from build123d import *

# Parameters (mm, degrees)
CYLINDER002_R         = 3.5
CYLINDER002_DEPTH     = 10
CYLINDER001_R         = 1.5
CYLINDER001_DEPTH     = 10
FUSION001_PITCH_ANGLE = 90
ARRAY001_COUNT        = 4
BOX002_W              = 6
BOX002_H              = 40
BOX002_DEPTH          = 25
CYLINDER_R            = 1.725
CYLINDER_DEPTH        = 10
ARRAY_X_COUNT         = 6
ARRAY_X_PITCH         = 20.333333
BOX_W                 = 194
BOX_H                 = 10
BOX_DEPTH             = 10
CHAMFER_SIZE          = 5


with BuildPart() as cylinder002:
    # Cylinder002 → Cylinder002 (new body)
    with BuildSketch(Plane(origin=(15, -5, 8), x_dir=(1, 0, 0), z_dir=(0, 0, 1))):
        Circle(CYLINDER002_R)
    extrude(amount=CYLINDER002_DEPTH)


with BuildPart() as cone:
    # Cone → Cone (revolve)
    with BuildSketch(Plane(origin=(15, -5, 6), x_dir=(1, 0, 0), z_dir=(0, -1, 0))):
        Polygon((0, 0), (1.5, 0), (3.5, 2), (0, 2), align=None)
    revolve(axis=Axis((15, -5, 6), (0, 0, 1)))


with BuildPart() as array001:
    # Cylinder001 → Cylinder001 (new body)
    with BuildSketch(Plane(origin=(15, -5, 0), x_dir=(1, 0, 0), z_dir=(0, 0, 1))):
        Circle(CYLINDER001_R)
    extrude(amount=CYLINDER001_DEPTH)

    # Fusion001: union Cylinder002, Cone
    add(cylinder002.part)
    add(cone.part)


with BuildPart() as array001_1:
    # Fusion001 pitch: moved
    add(array001.part.rotate(Axis((0, 0, 0), (0, 1, 0)), FUSION001_PITCH_ANGLE))


with BuildPart() as array001_2:
    # Fusion001 placement: moved
    add(array001_1.part.moved(Location((0, -10, 15))))

    # Array001: Array001 ×4 about axis
    array001_axis = Axis((0, 0, 0), (1, 0, 0))


with BuildPart() as array001_3:
    add(array001_2.part)
    for i in range(1, ARRAY001_COUNT):
        add(array001_2.part.rotate(array001_axis, i * 360 / ARRAY001_COUNT))


with BuildPart() as array001_4:
    # Array001 placement: moved
    add(array001_3.part.moved(Location((-6, 0, 0))))


with BuildPart() as cut001:
    # Box002 → Box002 (new body)
    with BuildSketch(Plane(origin=(0, -20, -20), x_dir=(1, 0, 0), z_dir=(0, 0, 1))):
        with Locations((3, 20)):
            Rectangle(BOX002_W, BOX002_H)
    extrude(amount=BOX002_DEPTH)

    # Cut001: cut Array001
    add(array001_4.part, mode=Mode.SUBTRACT)


with BuildPart() as cut001_1:
    # Cut001 placement: moved
    add(cut001.part.moved(Location((-6, 0, 0))))


with BuildPart() as array:
    # Cylinder → Cylinder (new body)
    with BuildSketch(Plane(origin=(185, 5, 0), x_dir=(1, 0, 0), z_dir=(0, 0, 1))):
        Circle(CYLINDER_R)
    extrude(amount=CYLINDER_DEPTH)

    # Array X: Array ×6


with BuildPart() as array_1:
    add(array.part)
    with Locations(*[(-i * ARRAY_X_PITCH, 0, 0) for i in range(1, ARRAY_X_COUNT)]):
        add(array.part)


with BuildPart() as chamfer_body:
    # Box → Box (new body)
    with BuildSketch(Plane.XY):
        with Locations((97, 5)):
            Rectangle(BOX_W, BOX_H)
    extrude(amount=BOX_DEPTH)

    # Cut: cut Array
    add(array_1.part, mode=Mode.SUBTRACT)


with BuildPart() as chamfer_body_1:
    # Cut placement: moved
    add(chamfer_body.part.moved(Location((0, -5, -5))))

    # Fusion: union Cut001
    add(cut001_1.part)

    # Chamfer
    chamfer_edges = [chamfer_body_1.edges().sort_by_distance(p)[0] for p in [
        (0, -5, 0),
        (0, 5, 0),
        (0, 0, -5),
    ]]
    chamfer(chamfer_edges, length=CHAMFER_SIZE)


solid = chamfer_body_1.part
For this review, take the finished solid that the model builds, in its own axes (mm). A direction names the side the tool comes from. Round coordinates to 2 decimals unless told otherwise and drop trailing zeros. Write each loop counter-clockwise with the first axis right and the second up, starting at its lowest first coordinate (ties: lowest second). Pieces come first, ordered by that corner, then holes. Notation, with made-up numbers: (20.5, -29) -> (24.5, -29) arc R20 ccw to (24.5, -24) -> close; hole circle Ø6 at (24, 35). An arc over 180 degrees is marked (long way). Put each result on its own line as item: value.
Q1. The part is to be moulded in two halves that separate along Y. For faces 1 (the flat face through (3, 7, -1)), 2 (the flat face through (86, 2, 5)), 3 (the cylindrical face through (142.964, -1.05, -0.07)), 4 (the flat face through (-3, -20, -8)), say which applies: released by +Y, released by -Y, zero draft, split by the parting line, or undercut.
Determined:
face 1: released by +Y
face 2: zero draft
face 3: undercut
face 4: released by -Y
Q2. Clearance check with flat-ended pins moving along their axes: pin 1 Ø5.5 at (x, y) = (185, 0) entering from -Z; pin 2 Ø6.5 at (y, z) = (15, 0) entering from +X; pin 3 Ø8 at (y, z) = (-5.5, -11.5) entering from +X. State where each tip first meets the part, or that it passes through.
Determined:
pin 1: stops at z = -5
pin 2: stops at x = -4.25
pin 3: stops at x = 2.5
Q3. Consider section C-C on x = 185. State the section outline as (y, z) points (3 decimals), and give its area (3 significant figures).
Determined:
outline: (-5, -5) -> (-1.725, -5) -> (-1.725, 5) -> (-5, 5) -> close; (1.725, -5) -> (5, -5) -> (5, 5) -> (1.725, 5) -> close
area: 65.5 mm^2
Q4. Consider section A-A on z = -15. State the section outline as (x, y) points, and give its area (3 significant figures).
Determined:
outline: (-6, -20) -> (0, -20) -> (0, -3.5) -> (-4, -3.5) -> (-6, -1.5) -> close; (-6, 1.5) -> (-4, 3.5) -> (0, 3.5) -> (0, 20) -> (-6, 20) -> close
area: 202 mm^2
Q5. Consider section B-B on y = -15. State the section outline as (x, z) points.
Determined:
outline: (-6, -20) -> (0, -20) -> (0, -3.5) -> (-4, -3.5) -> (-6, -1.5) -> close; (-6, 1.5) -> (-4, 3.5) -> (0, 3.5) -> (0, 5) -> (-6, 5) -> close
Q6. To check wall thickness, follow L1, parallel to Z at x = -2.75, y = 0; L2, parallel to Z at x = -2.1, y = -15; L3, parallel to Y at x = 185, z = 1.25 (3 decimals). State the ranges of each line that lie inside material, in increasing order. Write a range as [from, to].
Determined:
L1: z = [-20, -18.5], [-11.5, 5]
L2: z = [-20, -3.5], [3.5, 5]
L3: y = [-5, -1.725], [1.725, 5]
Q7. Machinability: for faces 5 (the flat face through (98, 0, -5)), 6 (the flat face through (-6, 0, -8)), 7 (the cylindrical face through (-2.028, -0.759, -18.417)), which of the approach directions +Z, -Z, +X, -X, +Y, -Y give a long, thin tool a straight path to every point of the face, cutting with its end or side? Answer none if there is none.
Determined:
face 5: -Z, +X, +Y, -Y
face 6: +Z, -Z, -X, +Y, -Y
face 7: +X
Q8. Consider section D-D on y = -7. State the section outline as (x, z) points.
Determined:
outline: (-6, -20) -> (0, -20) -> (0, -10) -> (3, -7) -> (3, 5) -> (-6, 5) -> close
